Geometry: final body of the model. Coordinates: model frame, mm. A direction names the side the tool comes from. Coordinates: 2 decimals unless noted, no trailing zeros. Order: outer loops, then holes, each group sorted by start corner. A loop starts at its lowest first (then second) coordinate and runs counter-clockwise, first axis right, second up. Notation, with made-up numbers: (-10, 37.5) -> (20, 37.5) arc R34 ccw to (20, 76.5) -> close; hole circle Ø8 at (27.25, -30.5). An arc over 180 degrees is marked (long way). Answer in a Markdown table with one row per item. Add a question column.
1) Ray query, line 1 (Z direction, x = 0.25, y = 1.5); line 2 (Z direction, x = -2.75, y = -3); line 3 (X direction, y = 0.25, z = -9.25). Return the intervals inside material, ascending. Write a range as from..to.
2) Contact query for flat-ended pins moving along their axis: P1, Ø2, axis at y = -0.5, z = 3, coming from the +X side; P2, Ø3, axis at y = 0.5, z = 3, coming from the -X side; P3, Ø3, axis at x = 2.5, z = -7, coming from the +Y side. Output: stop coordinate, or through.
3) Set-up query: faces 1 (the face through (-1.725, -3.045, 2.516)), 2 (the face through (3, 0.25, 3.4)), 3 (the face through (-1.8, 3, 2.5)), 4 (the face through (1.8, -3, 2.5)), 5 (the face through (1.725, 3.045, 2.516)). Return all of +Z, -Z, +X, -X, +Y, -Y with unobstructed straight access to the full face (end or side cutting, diameter ignored); none if empty.
4) Section query B-B on z = -12. Return the cut outline in (x, y), then the cut area to 3 significant figures.
5) Pull-direction query (X, two-part tool) for faces 6 (the face through (2, 1, 0)), 7 (the face through (0, -2, -10)), 8 (the face through (-3.5, 0, 3)), 9 (the face through (0, 0, 3)); classes: +X half, -X half, draft (parallel to the pull), parting line (faces both ways), or undercut.
```python
from build123d import *

# Parameters (mm, degrees)
HEAD_DEPTH         = 4
SHANK_SKETCH_R     = 2
SHANK_DEPTH        = 20
SKETCH6_R          = 2.625
HEAD_CUT_DEPTH     = 1
FILLET1_R          = 1
SKETCH8_W          = 3.5
SKETCH8_H          = 0.5
CUT_EXTRUDE3_DEPTH = 1


with BuildPart() as part:
    # Head Sketch → Head (new body)
    with BuildSketch(Plane.XY):
        Polygon((0, 4.041451884), (3.5, 2.020725942), (3.5, -2.020725942), (0, -4.041451884), (-3.5, -2.020725942), (-3.5, 2.020725942), align=None)
    extrude(amount=HEAD_DEPTH)

    # Shank Sketch → Shank (add)
    with BuildSketch(Plane.XY):
        Circle(SHANK_SKETCH_R)
    extrude(amount=-SHANK_DEPTH)

    # Sketch3 → Flange (revolve)
    with BuildSketch(Plane(origin=(0, 0, 0), x_dir=(-1, 0, 0), z_dir=(0, 1, 0)), mode=Mode.PRIVATE) as flange_sk:
        with BuildLine():
            Line((-5, 0), (0, 0))
            Line((0, 0), (0, 1.5))
            ThreePointArc((0, 1.5), (-2.562220765, 1.372207648), (-5.099009901, 0.99009901))
            ThreePointArc((-5.099009901, 0.99009901), (-5.497518595, 0.45024814), (-5, 0))
        make_face()
    revolve(flange_sk.sketch.rotate(Axis((0, 0, 0), (0, 0, 1)), 30), axis=Axis((0, 0, 0), (0, 0, 1)))

    # Sketch5 → Head Trim (revolve, cut)
    with BuildSketch(Plane(origin=(0, 0, 0), x_dir=(0, 0, -1), z_dir=(1, 0, 0)), mode=Mode.PRIVATE) as head_trim_sk:
        with BuildLine():
            Line((-4, -3.041451884), (-4, -4.041451884))
            Line((-4, -4.041451884), (-3, -4.041451884))
            ThreePointArc((-3, -4.041451884), (-3.707106781, -3.748558666), (-4, -3.041451884))
        make_face()
    revolve(head_trim_sk.sketch.rotate(Axis((0, 0, 15.085599173), (0, 0, -1)), 90), axis=Axis((0, 0, 15.085599173), (0, 0, -1)), mode=Mode.SUBTRACT)

    # Sketch6 → Head Cut (cut)
    with BuildSketch(Plane.XY.offset(4)):
        Circle(SKETCH6_R)
    extrude(amount=-HEAD_CUT_DEPTH, mode=Mode.SUBTRACT)

    # Fillet1
    fillet1_edges = [part.edges().sort_by_distance(p)[0] for p in [
        (-2.625, 0, 3),
    ]]
    fillet(fillet1_edges, radius=FILLET1_R - 0.0001)  # a hair under: the kernel refuses the full size

    # Sketch8 → Cut-Extrude3 (cut)
    with BuildSketch(Plane.XY.offset(4)):
        with Locations((1.75, 0)):
            Rectangle(SKETCH8_W, SKETCH8_H)
    extrude(amount=-CUT_EXTRUDE3_DEPTH, mode=Mode.SUBTRACT)


solid = part.part
```
Result:
| question | item | result |
|---|---|---|
| 1 | line 1 | -20..3 |
| 1 | line 2 | 0..1.18 |
| 1 | line 3 | -1.98..1.98 |
| 2 | P1 | x = 3.5 |
| 2 | P2 | x = -3.5 |
| 2 | P3 | y = 1.73 |
| 3 | face 1 | +Z, -X, -Y |
| 3 | face 2 | +Z, +X |
| 3 | face 3 | +Z, -X, +Y |
| 3 | face 4 | +Z, +X, -Y |
| 3 | face 5 | +Z, +X, +Y |
| 4 | outline | circle Ø4 at (0, 0) |
| 4 | area | 12.6 mm2 |
| 5 | face 6 | draft |
| 5 | face 7 | parting line |
| 5 | face 8 | -X half |
| 5 | face 9 | undercut |
